Geometry: final body of the model. Coordinates: model frame, mm. Face numbers are marked on the shaded views. A direction names the side the tool comes from. Give positions to 0.01 mm unless a question says otherwise; leave off trailing zeros. Write each loop counter-clockwise with the first axis right and the second up, starting at its lowest first coordinate (ties: lowest second). Pieces come first, ordered by that corner, then holes. Notation, with made-up numbers: M -1.75,15.25 L 21.25,15.25 A13 ccw 21.25,26.25 Z; hole C 75.5,-2 d4. An arc over 180 degrees is marked long. Use a Markdown table: item, result. Add a question column.
1) Line query: line 1 (Y direction, x = 45.72, z = 3.75) (1 decimal); line 2 (Y direction, x = 7.62, z = 3) (1 decimal); line 3 (X direction, y = 21, z = 3) (3 decimals). Output: solid intervals per line, ascending.
2) Set-up query: the marked faces 1, 2 and 3. Return all of +Z, -Z, +X, -X, +Y, -Y with unobstructed straight access to the full face (end or side cutting, diameter ignored); none if empty.
3) Pin query (flat end, axial travel): pin 1 (1.5 mm diameter, centred on x = 35, z = 5.5, fed in from +Y) (3 decimals); pin 2 (1.9 mm diameter, centred on x = 7.62, y = 66.04, fed in from -Z); pin 3 (1.9 mm diameter, centred on x = 1.5, z = 2.5, fed in from -Y) (3 decimals); pin 4 (2 mm diameter, centred on x = 52, z = 4, fed in from +Y). Return the tip coordinate at first contact, or that it passes through.
4) Draft query along X for the marked faces 4, 5, 6 and 7. Return one class per face: +X half, -X half, draft (parallel to the pull), parting line (faces both ways), or undercut.
5) Section B-B on y = 60. Return the cut outline in (x, z) (3 decimals).
6) Section A-A on x = 45.72. State how many separate pieces and enclosed holes the cut face has, then the cut area to 3 significant figures.
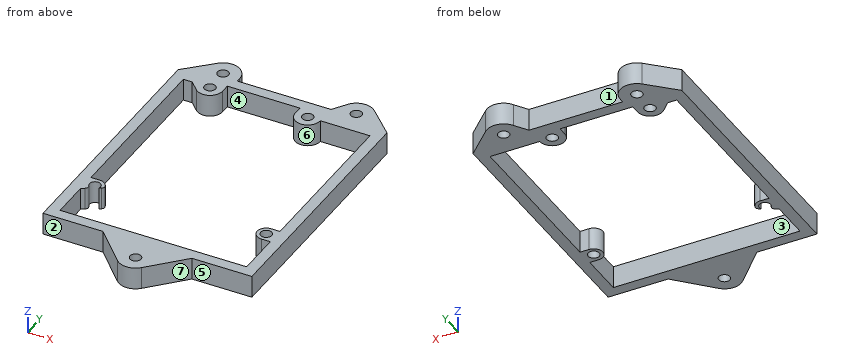
```python
from build123d import *

# Parameters (mm, degrees)
SKETCH1_R           = 1.5875
BOSS_EXTRUDE1_DEPTH = 6.35
FILLET1_R           = 1


with BuildPart() as part:
    # Sketch1 → Boss-Extrude1 (new body)
    with BuildSketch(Plane.XY):
        with BuildLine():
            Line((13.97, -3.175), (23.234773085, -12.823578829))
            ThreePointArc((23.234773085, -12.823578829), (26.67, -14.2875), (30.105226915, -12.823578829))
            Line((30.105226915, -12.823578829), (39.37, -3.175))
            Line((39.37, -3.175), (56.515, -3.175))
            Line((56.515, -3.175), (56.515, 69.215))
            Line((56.515, 69.215), (49.029740814, 76.449473973))
            ThreePointArc((49.029740814, 76.449473973), (45.054787809, 77.740813715), (41.592139899, 75.400326764))
            Line((41.592139899, 75.400326764), (39.161128061, 71.755))
            Line((39.161128061, 71.755), (12.3825, 71.755))
            Line((12.3825, 71.755), (12.3825, 73.025))
            ThreePointArc((12.3825, 73.025), (9.479941615, 77.409292809), (4.310259186, 76.449473973))
            Line((4.310259186, 76.449473973), (-3.175, 69.215))
            Line((-3.175, 69.215), (-3.175, -3.175))
            Line((-3.175, -3.175), (13.97, -3.175))
        make_face()
        with Locations((35.56, 66.04)):
            Circle(SKETCH1_R, mode=Mode.SUBTRACT)
        with Locations((7.62, 66.04)):
            Circle(SKETCH1_R, mode=Mode.SUBTRACT)
        with Locations((50.8, 15.24)):
            Circle(SKETCH1_R, mode=Mode.SUBTRACT)
        with Locations((26.67, -9.525)):
            Circle(SKETCH1_R, mode=Mode.SUBTRACT)
        with Locations((45.72, 73.025)):
            Circle(SKETCH1_R, mode=Mode.SUBTRACT)
        with Locations((7.62, 73.025)):
            Circle(SKETCH1_R, mode=Mode.SUBTRACT)
        with BuildLine():
            Line((53.34, 66.04), (53.34, 17.8275))
            Line((53.34, 17.8275), (50.8, 17.8275))
            ThreePointArc((50.8, 17.8275), (48.2125, 15.24), (50.8, 12.6525))
            Line((50.8, 12.6525), (53.34, 12.6525))
            Line((53.34, 12.6525), (53.34, 0))
            Line((53.34, 0), (0, 0))
            Line((0, 0), (0, 11.093834149))
            Line((0, 11.093834149), (2.323755448, 12.397297058))
            ThreePointArc((2.323755448, 12.397297058), (1.763362672, 15.354554336), (3.994811275, 13.334641515))
            Line((3.994811275, 13.334641515), (5.1275, 13.97))
            ThreePointArc((5.1275, 13.97), (4.369638796, 15.799638796), (2.54, 16.5575))
            Line((2.54, 16.5575), (0, 16.5575))
            Line((0, 16.5575), (0, 66.04))
            Line((0, 66.04), (2.54, 66.04))
            Line((2.54, 66.04), (5.08, 63.506513025))
            ThreePointArc((5.08, 63.506513025), (8.990749111, 62.724701654), (11.2075, 66.04))
            Line((11.2075, 66.04), (11.2075, 68.58))
            Line((11.2075, 68.58), (31.9725, 68.58))
            Line((31.9725, 68.58), (31.9725, 66.04))
            ThreePointArc((31.9725, 66.04), (35.56, 62.4525), (39.1475, 66.04))
            Line((39.1475, 66.04), (40.386, 66.04))
            Line((40.386, 66.04), (53.34, 66.04))
        make_face(mode=Mode.SUBTRACT)
    extrude(amount=BOSS_EXTRUDE1_DEPTH)

    # Fillet1
    fillet1_edges = [part.edges().sort_by_distance(p)[0] for p in [
        (5.1275, 13.97, 3.175),
        (2.323755448, 12.397297058, 3.175),
    ]]
    fillet(fillet1_edges, radius=FILLET1_R)


solid = part.part
```
Found:
| question | item | result |
|---|---|---|
| 1 | line 1 | -3.2 to 0, 66 to 71.4, 74.6 to 77.8 |
| 1 | line 2 | -3.2 to 0, 62.5 to 64.5, 67.6 to 71.4, 74.6 to 77.8 |
| 1 | line 3 | -3.175 to 0, 53.34 to 56.515 |
| 2 | face 1 | +Z, -Z, +Y |
| 2 | face 2 | +Z, -Z, -X, -Y |
| 2 | face 3 | +Z, -Z |
| 3 | pin 1 | y = 71.755 |
| 3 | pin 2 | through |
| 3 | pin 3 | y = -3.175 |
| 3 | pin 4 | y = 74.55 |
| 4 | face 4 | undercut |
| 4 | face 5 | draft |
| 4 | face 6 | undercut |
| 4 | face 7 | +X half |
| 5 | outline | M -3.175,0 L 0,0 L 0,6.35 L -3.175,6.35 Z; M 53.34,0 L 56.515,0 L 56.515,6.35 L 53.34,6.35 Z |
| 6 | separate pieces | 3 |
| 6 | enclosed holes | 0 |
| 6 | area | 74.6 mm² |
